```python
from build123d import *

# Parameters (mm, degrees)
SKETCH1_W           = 125
SKETCH1_H           = 60
SKETCH1_W_2         = 4
SKETCH1_H_2         = 8
BOSS_EXTRUDE1_DEPTH = 4
BOSS_EXTRUDE2_DEPTH = 4


with BuildPart() as part:
    # Sketch1 → Boss-Extrude1 (new body)
    with BuildSketch(Plane.XY):
        with Locations((-6, 0)):
            Rectangle(SKETCH1_W, SKETCH1_H)
        with Locations((-36.5, 21)):
            Rectangle(SKETCH1_W_2, SKETCH1_H_2, mode=Mode.SUBTRACT)
        with Locations((24.5, 21)):
            Rectangle(SKETCH1_W_2, SKETCH1_H_2, mode=Mode.SUBTRACT)
        with Locations((24.5, -21)):
            Rectangle(SKETCH1_W_2, SKETCH1_H_2, mode=Mode.SUBTRACT)
        with Locations((-24.5, 21)):
            Rectangle(SKETCH1_W_2, SKETCH1_H_2, mode=Mode.SUBTRACT)
        with Locations((-24.5, -21)):
            Rectangle(SKETCH1_W_2, SKETCH1_H_2, mode=Mode.SUBTRACT)
        with Locations((49.5, 21)):
            Rectangle(SKETCH1_W_2, SKETCH1_H_2, mode=Mode.SUBTRACT)
        with Locations((49.5, -21)):
            Rectangle(SKETCH1_W_2, SKETCH1_H_2, mode=Mode.SUBTRACT)
        with Locations((-36.5, -21)):
            Rectangle(SKETCH1_W_2, SKETCH1_H_2, mode=Mode.SUBTRACT)
        with Locations((-61.5, 21)):
            Rectangle(SKETCH1_W_2, SKETCH1_H_2, mode=Mode.SUBTRACT)
        with Locations((-61.5, -21)):
            Rectangle(SKETCH1_W_2, SKETCH1_H_2, mode=Mode.SUBTRACT)
    extrude(amount=BOSS_EXTRUDE1_DEPTH)

    # Sketch2 → Boss-Extrude2 (add)
    with BuildSketch(Plane.XY):
        Polygon((-68.5, 30), (-68.5, 55), (-53.5, 55), (-39.357864376, 40.857864376), (27.357864376, 40.857864376), (41.5, 55), (56.5, 55), (56.5, 30), align=None)
    extrude(amount=BOSS_EXTRUDE2_DEPTH)


solid = part.part
```
Part model, mm, in its own coordinate system. Give positions to 0.01 mm unless a question says otherwise; leave off trailing zeros. Write each loop counter-clockwise with the first axis right and the second up, starting at its lowest first coordinate (ties: lowest second). Pieces come first, ordered by that corner, then holes. Notation, with made-up numbers: (-5.5, 33.25) -> (44.5, 33.25) arc R17 ccw to (44.5, 66.25) -> close; hole circle Ø10 at (22, -39.75). An arc over 180 degrees is marked (long way). Put each result on its own line as item: value. Start each with the question number.
Item 1: Cut at D-D (x = -12.5). List the corners of the cut face in (y, z).
Item 2: Pull direction Y, two halves, no side cores. Call faces 1 (the face through (-5, 4, 0)), 2 (the face through (-25, -17, 2)): pulls with the +Y half, pulls with the -Y half, needs draft (parallel to the pull), parting line crosses it, or undercut.
Item 3: Cut at C-C (z = 1.2). State how many separate pieces and enclosed holes the cut face has, then the cut area to 3 significant figures.
Item 4: Cut at A-A (y = -23). List the corners of the cut face in (x, z), then the cut area to 3 significant figures.
Item 5: Wall check: L1, parallel to X at y = 20, z = 3.6; L2, parallel to Y at x = 49, z = 0.4; L3, parallel to Y at x = -25, z = 2.45. Give the ranges that are in metal, low to high. Write a range as [from, to].
Item 6: Cut at B-B (x = -49). List the corners of the cut face in (y, z), then the cut area to 3 significant figures.
Item 7: Pin check, flat tip, straight feed: pin 1 Ø1.5 at (x, z) = (-19.5, 2) entering from +Y. Stop position of the tip, or through.
Answer list:
1. outline: (-30, 0) -> (40.86, 0) -> (40.86, 4) -> (-30, 4) -> close
2. face 1: needs draft
2. face 2: undercut
3. separate pieces: 1
3. enclosed holes: 10
3. area: 9,160 mm2
4. outline: (-68.5, 0) -> (-63.5, 0) -> (-63.5, 4) -> (-68.5, 4) -> close; (-59.5, 0) -> (-38.5, 0) -> (-38.5, 4) -> (-59.5, 4) -> close; (-34.5, 0) -> (-26.5, 0) -> (-26.5, 4) -> (-34.5, 4) -> close; (-22.5, 0) -> (22.5, 0) -> (22.5, 4) -> (-22.5, 4) -> close; (26.5, 0) -> (47.5, 0) -> (47.5, 4) -> (26.5, 4) -> close; (51.5, 0) -> (56.5, 0) -> (56.5, 4) -> (51.5, 4) -> close
4. area: 420 mm2
5. L1: x = [-68.5, -63.5], [-59.5, -38.5], [-34.5, -26.5], [-22.5, 22.5], [26.5, 47.5], [51.5, 56.5]
5. L2: y = [-30, -25], [-17, 17], [25, 55]
5. L3: y = [-30, -25], [-17, 17], [25, 40.86]
6. outline: (-30, 0) -> (50.5, 0) -> (50.5, 4) -> (-30, 4) -> close
6. area: 322 mm2
7. pin 1: stops at y = 40.86
